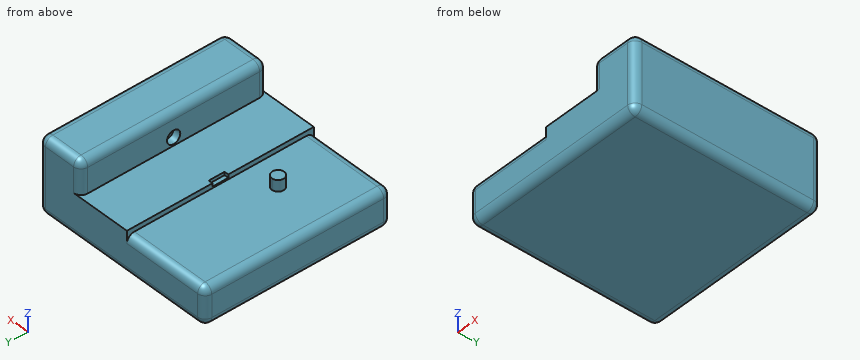
```python
from build123d import *

# Parameters (mm, degrees)
F0_W      = 100
F0_H      = 100
F1_DEPTH  = 10
F3_W      = 25
F3_H      = 10.365
F4_DEPTH  = 100
F6_DEPTH  = 4.045
F7_DEPTH  = 28.235
F9_DEPTH  = 2.25
F11_DEPTH = 5.97
F12_R     = 4
F13_W     = 2.25
F13_H     = 8.4769393061
F14_DEPTH = 1.73


with BuildPart() as f1:
    # F0 (on Top) → F1 (new body, symmetric)
    with BuildSketch(Plane.XY):
        Rectangle(F0_W, F0_H)
    extrude(amount=F1_DEPTH, both=True)

    # F3 (on face) → F4 (join)
    with BuildSketch(Plane.XZ.offset(50)):
        Polygon((25, 10), (50, 10), (50, 19.635), (25, 19.635), (25, 16.095), (25, 12.555), align=None)
        with Locations((37.5, 24.8175)):
            Rectangle(F3_W, F3_H)
    extrude(amount=-F4_DEPTH)

    # F5 (on face) → F6 (cut)
    with BuildSketch(Plane(origin=(25, 0, 0), x_dir=(0, -1, 0), z_dir=(-1, 0, 0))):
        with BuildLine():
            ThreePointArc((3.54, 16.935), (-2.5031580054, 19.4381580054), (0, 13.395))
            ThreePointArc((0, 13.395), (2.5031580054, 14.4318419946), (3.54, 16.935))
        make_face()
    extrude(amount=-F6_DEPTH, mode=Mode.SUBTRACT)

    # F5 (on face) → F7 (join)
    with BuildSketch(Plane(origin=(25, 0, 0), x_dir=(0, -1, 0), z_dir=(-1, 0, 0))):
        Polygon((0, 10), (50, 10), (50, 11.715), (50, 12.555), (0, 12.555), align=None)
        Polygon((-50, 10), (0, 10), (0, 12.555), (-50, 12.555), (-50, 11.715), align=None)
    extrude(amount=F7_DEPTH)

    # F8 (on face) → F9 (cut)
    with BuildSketch(Plane(origin=(-3.235, 0, 0), x_dir=(0, -1, 0), z_dir=(-1, 0, 0))):
        with BuildLine():
            Line((0, 10.84), (0, 12.555))
            Line((0, 12.555), (-4.2384696531, 12.555))
            ThreePointArc((-4.2384696531, 12.555), (-2.286145774, 11.284994469), (0, 10.84))
        make_face()
        with BuildLine():
            Line((4.2384696531, 12.555), (0, 12.555))
            Line((0, 12.555), (0, 10.84))
            ThreePointArc((0, 10.84), (2.286145774, 11.284994469), (4.2384696531, 12.555))
        make_face()
    extrude(amount=-F9_DEPTH, mode=Mode.SUBTRACT)

    # F10 (on face) → F11 (join)
    with BuildSketch(Plane.XY.offset(10)):
        with BuildLine():
            ThreePointArc((-16.665, -16.13), (-17.613974029, -13.838974029), (-19.905, -12.89))
            ThreePointArc((-19.905, -12.89), (-22.196025971, -18.421025971), (-16.665, -16.13))
        make_face()
    extrude(amount=F11_DEPTH)

    # F12
    f12_edges = [f1.edges().sort_by_distance(p)[0] for p in [
        (25, 0, 30),
        (50, 0, 30),
        (-50, 0, 10),
        (-50, 0, -10),
        (50, 0, -10),
        (25, -50, 21.2775),
        (37.5, -50, 30),
        (50, -50, 10),
        (0, -50, -10),
        (-50, -50, 0),
        (-50, 50, 0),
        (-26.6175, 50, 10),
        (25, 50, 21.2775),
        (37.5, 50, 30),
        (50, 50, 10),
        (0, 50, -10),
        (-26.6175, -50, 10),
    ]]
    fillet(f12_edges, radius=F12_R)

    # F13 (on face) → F14 (cut)
    with BuildSketch(Plane.XY.offset(12.555)):
        with Locations((-2.11, 0)):
            Rectangle(F13_W, F13_H)
    extrude(amount=-F14_DEPTH, mode=Mode.SUBTRACT)


solid = f1.part
```
The model under review builds one solid part; all positions refer to its coordinate system, in mm. Give positions to 0.01 mm unless a question says otherwise; leave off trailing zeros. Loops run counter-clockwise (first coordinate to the right, second up) from the corner with the lowest first, then second, coordinate; pieces in that order, holes last. Notation, with made-up numbers: (47.5, 37.25) - (91.5, 37.25) arc R14 ccw to (91.5, 52.25) - close; hole circle Ø4 at (15.5, -11). An arc over 180 degrees is marked (long way). Answer as a JSON object with one key per item and string values.
Q1. Add section A-A on y = 37. State the section outline as (x, z) points (3 decimals), plus the area to 3 significant figures.
Worked out:
{"outline": "(-50, -6) arc R4 ccw to (-46, -10) - (46, -10) arc R4 ccw to (50, -6) - (50, 26) arc R4 ccw to (46, 30) - (29, 30) arc R4 ccw to (25, 26) - (25, 12.555) - (-3.235, 12.555) - (-3.235, 10) - (-46, 10) arc R4 ccw to (-50, 6) - close", "area": "2,550 mm^2"}
Q2. Insertion check: pin 1 (3 mm diameter, centred on y = -29, z = 20, fed in from -X); pin 2 (1.9 mm diameter, centred on y = 1, z = 12, fed in from -X) (3 decimals); pin 3 (5.5 mm diameter, centred on y = 0.5, z = 17, fed in from -X) (3 decimals). Each pin has a flat end and moves straight along its axis. Give the tip position at first contact, or say it passes through.
Worked out:
{"pin 1": "stops at x = 25", "pin 2": "stops at x = -0.985", "pin 3": "stops at x = 29.045"}
Q3. Add section D-D on y = 0. State the section outline as (x, z) points (3 decimals).
Worked out:
{"outline": "(-50, -6) arc R4 ccw to (-46, -10) - (46, -10) arc R4 ccw to (50, -6) - (50, 26) arc R4 ccw to (46, 30) - (29, 30) arc R4 ccw to (25, 26) - (25, 20.475) - (29.045, 20.475) - (29.045, 13.395) - (25, 13.395) - (25, 12.555) - (-0.985, 12.555) - (-0.985, 10.825) - (-3.235, 10.825) - (-3.235, 10) - (-46, 10) arc R4 ccw to (-50, 6) - close"}
Q4. Add section C-C on z = 22. State the section outline as (x, y) points.
Worked out:
{"outline": "(25, -46) arc R4 ccw to (29, -50) - (46, -50) arc R4 ccw to (50, -46) - (50, 46) arc R4 ccw to (46, 50) - (29, 50) arc R4 ccw to (25, 46) - close"}
Q5. To check wall thickness, follow line 1 along Z through (x, y) = (-46, -15); line 2 along X through (y, z) = (-28.5, 13); line 3 along Z through (x, y) = (-19, -14.5). State the ranges of each line that lie inside material, in increasing order.
Worked out:
{"line 1": "z = -10 to 10", "line 2": "x = 25 to 50", "line 3": "z = -10 to 15.97"}
Q6. Add section B-B on x = 3.5. State the section outline as (y, z) points (3 decimals), plus the area to 3 significant figures.
Worked out:
{"outline": "(-50, -6) arc R4 ccw to (-46, -10) - (46, -10) arc R4 ccw to (50, -6) - (50, 12.555) - (-50, 12.555) - close", "area": "2,250 mm^2"}
